Geometry: final body of the model. Coordinates: model frame, mm. A direction names the side the tool comes from. Coordinates: 2 decimals unless noted, no trailing zeros. Write each loop counter-clockwise with the first axis right and the second up, starting at its lowest first coordinate (ties: lowest second). Pieces come first, ordered by that corner, then holes. Notation, with made-up numbers: (10, 83.5) - (69, 83.5) arc R17 ccw to (69, 105.5) - close; hole circle Ø4 at (62.25, -11). An arc over 180 degrees is marked (long way). Answer as a JSON object with one key per item and string values. Group by question number.
Item 1: Set-up query: faces 4 (the flat face through (27.5, 5, 0)), 5 (the flat face through (-37.5, 3, 1)). Return all of +Z, -Z, +X, -X, +Y, -Y with unobstructed straight access to the full face (end or side cutting, diameter ignored); none if empty.
Item 2: Section A-A on z = -25. Return loops of the section in (x, y), and give its area (3 significant figures).
Item 3: First-contact query: pin 1 Ø4 at (y, z) = (5.5, 1) entering from +X; pin 2 Ø5 at (x, z) = (-27.5, 25) entering from +Y. Flat tips, straight axial feed; report the tip coordinate or a pass-through.
Item 4: Section B-B on x = -27.5. Return loops of the section in (y, z).
Item 5: Line query: line 1 along X through (y, z) = (3, -25); line 2 along Z through (x, y) = (-2.5, 2.5); line 3 along Z through (x, y) = (-29.5, 4.5). Output: solid intervals per line, ascending. Write a range as from..to.
Item 6: Mould query, pull axis Y, two halves, no side actions, for faces 1 (the cylindrical face through (-3.172, 3.549, -21.974)), 2 (the flat face through (33, 3.464, 0)), 3 (the flat face through (1, 7, 1)). Classes: pulls with the +Y half, pulls with the -Y half, needs draft (parallel to the pull), parting line crosses it, or undercut.
Autodesk Inventor part; units mm, degrees
ref_plane "YZ Plane" through (0, 0, 0) normal (1, 0, 0) x (0, 1, 0)
ref_plane "XZ Plane" through (0, 0, 0) normal (0, 1, 0) x (-1, 0, 0)
ref_plane "XY Plane" through (0, 0, 0) normal (0, 0, 1) x (1, 0, 0)
sketch "Sketch1" plane through (0, 0, 0) normal (0, 1, 0) x (-1, 0, 0)
  line L0 (-37.5, 37.5) -> (37.5, 37.5)
  line L1 (37.5, 37.5) -> (37.5, -37.5)
  line L2 (37.5, -37.5) -> (-37.5, -37.5)
  line L3 (-37.5, -37.5) -> (-37.5, 37.5)
  line L4 (-37.5, 37.5) -> (37.5, -37.5) construction
  line L5 (37.5, 37.5) -> (-37.5, -37.5) construction
  point P0 (0, 0)
  dimension "d0" = 75
  dimension "d1" = 75
extrude "Extrusion1" add sketch "Sketch1" along normal blind 7
sketch "Sketch2" plane through (0, 7, 0) normal (0, 1, 0) x (1, 0, 0)
  circle A0 centre (-27.5, -25) radius 3.1
  line L0 (-37.5, -37.5) -> (37.5, -37.5)
  line L1 (37.5, -37.5) -> (37.5, 37.5)
  circle A1 centre (-2.5, -25) radius 3.1
  point P0 (0, 0)
  dimension "d4" = 6.2
  dimension "d5" = 12.5
  dimension "d6" = 65
  dimension "d19" = 6.2
  dimension "d20" = 12.5
  dimension "d21" = 40
extrude "Extrusion2" cut sketch "Sketch2" against normal through all
mirror "Mirror1" about plane through (0, 0, 0) normal (0, 0, 1) of "Extrusion2"
sketch "Sketch3" plane through (37.5, 0, 37.5) normal (1, 0, 0) x (0, 0, -1)
  line L0 (0, 7) -> (75, 7)
  line L1 (33.5, 7) -> (29.9645, 3.4645)
  line L2 (33.5, 7) -> (38.5, 7) construction
  line L3 (33.5, 7) -> (41.5, 7)
  line L4 (33.5, 7) -> (41.5, 7) construction
  line L5 (41.5, 7) -> (45.0355, 3.4645)
  line L6 (45.0355, 3.4645) -> (29.9645, 3.4645)
  point P0 (37.5, 0)
  dimension "d9" = 5
  dimension "d10" = 135
  dimension "d11" = 33.5
  dimension "d12" = 8
  dimension "d13" = 0
  dimension "d14" = 5
  dimension "d15" = 135
extrude "Extrusion3" cut sketch "Sketch3" against normal blind 10
fillet "Fillet1" radius 1 3 edges at (0, 7, -37.5) (-37.5, 7, 0) (0, 7, 37.5)
properties part number "Dovetail_holder_V3"
Checks:
{
 "1": {"face 4": "+X", "face 5": "+Z, -Z, -X, +Y, -Y"},
 "2": {"outline": "(-37.5, 0) - (-30.6, 0) - (-30.6, 7) - (-36.5, 7) arc R1 ccw to (-37.5, 6) - close; (-24.4, 0) - (-5.6, 0) - (-5.6, 7) - (-24.4, 7) - close; (0.6, 0) - (37.5, 0) - (37.5, 7) - (0.6, 7) - close", "area": "438 mm^2"},
 "3": {"pin 1": "x = 27.5", "pin 2": "through"},
 "4": {"outline": "(0, -37.5) - (6, -37.5) arc R1 ccw to (7, -36.5) - (7, -28.1) - (0, -28.1) - close; (0, -21.9) - (7, -21.9) - (7, 21.9) - (0, 21.9) - close; (0, 28.1) - (7, 28.1) - (7, 36.5) arc R1 ccw to (6, 37.5) - (0, 37.5) - close"},
 "5": {"line 1": "-37.5..-30.6, -24.4..-5.6, 0.6..37.5", "line 2": "-37.5..-28.1, -21.9..21.9, 28.1..37.5", "line 3": "-37.5..-27.37, -22.63..22.63, 27.37..37.5"},
 "6": {"face 1": "needs draft", "face 2": "undercut", "face 3": "pulls with the +Y half"}
}
